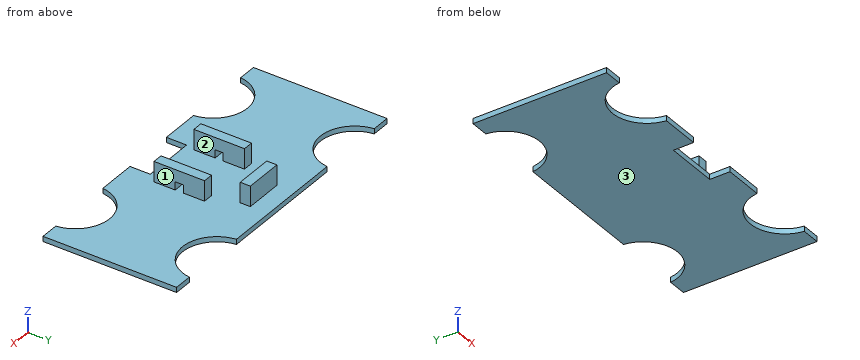
```python
from build123d import *

# Parameters (mm, degrees)
BOSS_EXTRUDE1_DEPTH = 2.54
SKETCH2_W           = 26.0160991
SKETCH2_H           = 10
CUT_EXTRUDE1_DEPTH  = 2.54
SKETCH6_W           = 5
SKETCH6_H           = 25
BOSS_EXTRUDE2_DEPTH = 10
SKETCH6_3_W         = 19
SKETCH6_3_H         = 5
BOSS_EXTRUDE3_DEPTH = 10
SKETCH6_4_W         = 5
SKETCH6_4_H         = 25
BOSS_EXTRUDE4_DEPTH = 10
SKETCH9_W           = 4
SKETCH9_H           = 2
CUT_EXTRUDE3_DEPTH  = 99.671329208


with BuildPart() as part:
    # Sketch1 → Boss-Extrude1 (new body)
    with BuildSketch(Plane.XY):
        with BuildLine():
            Line((-32.468057, 32.999999883), (-13, 32.999999883))
            Line((-13, 32.999999883), (13, 32.999999883))
            Line((13, 32.999999883), (32.468057241, 32.999999883))
            ThreePointArc((32.468057241, 32.999999883), (49.350000777, 18.000000029), (66.231944118, 33.000000103))
            Line((66.231944118, 33.000000103), (75.350000118, 33.000000103))
            Line((75.350000118, 33.000000103), (75.350000118, -32.999998949))
            Line((75.350000118, -32.999998949), (66.231943, -32.999998949))
            ThreePointArc((66.231943, -32.999998949), (49.349999056, -17.999999409), (32.468056, -32.999999949))
            Line((32.468056, -32.999999949), (13, -32.999999949))
            Line((13, -32.999999949), (-12.999999882, -32.999999949))
            Line((-12.999999882, -32.999999949), (-32.468057, -32.999999117))
            ThreePointArc((-32.468057, -32.999999117), (-49.350000944, -17.999999578), (-66.231944, -33.000000117))
            Line((-66.231944, -33.000000117), (-75.35, -33.000000117))
            Line((-75.35, -33.000000117), (-75.35, 32.999999883))
            Line((-75.35, 32.999999883), (-66.231944, 32.999999883))
            ThreePointArc((-66.231944, 32.999999883), (-49.3500005, 17.999999403), (-32.468057, 32.999999883))
        make_face()
    extrude(amount=BOSS_EXTRUDE1_DEPTH)

    # Sketch2 → Cut-Extrude1 (cut)
    with BuildSketch(Plane.XY.offset(2.54)):
        with Locations((0.008049668, -27.999999949)):
            Rectangle(SKETCH2_W, SKETCH2_H)
    extrude(amount=-CUT_EXTRUDE1_DEPTH, mode=Mode.SUBTRACT)

    # Sketch6 → Boss-Extrude2 (add)
    with BuildSketch(Plane.XY.offset(2.54)):
        with Locations((-14.289999882, -6.066775281)):
            Rectangle(SKETCH6_W, SKETCH6_H)
    extrude(amount=BOSS_EXTRUDE2_DEPTH)

    # Sketch6_3 → Boss-Extrude3 (add)
    with BuildSketch(Plane.XY.offset(2.54)):
        with Locations((0.010000118, 21.520000051)):
            Rectangle(SKETCH6_3_W, SKETCH6_3_H)
    extrude(amount=BOSS_EXTRUDE3_DEPTH)

    # Sketch6_4 → Boss-Extrude4 (add)
    with BuildSketch(Plane.XY.offset(2.54)):
        with Locations((14.310000118, -6.066775281)):
            Rectangle(SKETCH6_4_W, SKETCH6_4_H)
    extrude(amount=BOSS_EXTRUDE4_DEPTH)

    # Sketch9 → Cut-Extrude3 (cut, through all)
    with BuildSketch(Plane.ZY.offset(16.789999882)):
        with Locations((4.54, -5.066775281)):
            Rectangle(SKETCH9_W, SKETCH9_H)
        with Locations((4.54, -7.066775281)):
            Rectangle(SKETCH9_W, SKETCH9_H)
    extrude(amount=-CUT_EXTRUDE3_DEPTH, mode=Mode.SUBTRACT)


solid = part.part
```
CAD build for the part. Positions are in the model's coordinates, mm. Face numbers are marked on the shaded views. Coordinates: 2 decimals unless noted, no trailing zeros. Write each loop counter-clockwise with the first axis right and the second up, starting at its lowest first coordinate (ties: lowest second). Pieces come first, ordered by that corner, then holes.
(1) Cut at A-A, the plane z = 10.75. List the corners of the cut face in (x, y), and give its area (3 significant figures).
(2) Two-plate mould, pull along X, no slides. Class the marked faces 1, 2 and 3: +X half, -X half, draft (parallel to the pull), parting line (faces both ways), or undercut.
(3) Cut at D-D, the plane z = 4.5. List the corners of the cut face in (x, y), and give its area (3 significant figures).
(4) Flat gauge pins, fed straight in: pin 1 (1.5 mm diameter, centred on x = -15, z = 7, fed in from -Y); pin 2 (5 mm diameter, centred on y = -5, z = 6, fed in from -X); pin 3 (1.5 mm diameter, centred on x = -8.5, y = -15.5, fed in from +Z). Where does each tip first touch, or does it go through?
(5) Cut at B-B, the plane x = 15. List the corners of the cut face in (y, z), and give its area (3 significant figures).
(6) Drill centre lines: probe 1 along X at (y, z) = (-1, 8.25); probe 2 along Z at (x, y) = (27, -29); probe 3 along X at (y, z) = (22.5, 5.75). Where is each one in solid material? Low to high.
(7) Cut at C-C, the plane y = -15.5. List the corners of the cut face in (x, z).
Geometry says:
1. outline: (-16.79, -18.57) - (-11.79, -18.57) - (-11.79, 6.43) - (-16.79, 6.43) - close; (-9.49, 19.02) - (9.51, 19.02) - (9.51, 24.02) - (-9.49, 24.02) - close; (11.81, -18.57) - (16.81, -18.57) - (16.81, 6.43) - (11.81, 6.43) - close
1. area: 345 mm2
2. face 1: +X half
2. face 2: undercut
2. face 3: draft
3. outline: (-16.79, -18.57) - (-11.79, -18.57) - (-11.79, -8.07) - (-16.79, -8.07) - close; (-16.79, -4.07) - (-11.79, -4.07) - (-11.79, 6.43) - (-16.79, 6.43) - close; (-9.49, 19.02) - (9.51, 19.02) - (9.51, 24.02) - (-9.49, 24.02) - close; (11.81, -18.57) - (16.81, -18.57) - (16.81, -8.07) - (11.81, -8.07) - close; (11.81, -4.07) - (16.81, -4.07) - (16.81, 6.43) - (11.81, 6.43) - close
3. area: 305 mm2
4. pin 1: stops at y = -18.57
4. pin 2: stops at x = -16.79
4. pin 3: stops at z = 2.54
5. outline: (-33, 0) - (33, 0) - (33, 2.54) - (6.43, 2.54) - (6.43, 12.54) - (-18.57, 12.54) - (-18.57, 2.54) - (-33, 2.54) - close; hole (-8.07, 2.54) - (-4.07, 2.54) - (-4.07, 6.54) - (-8.07, 6.54) - close
5. area: 402 mm2
6. probe 1: x = -16.79 to -11.79, 11.81 to 16.81
6. probe 2: z = 0 to 2.54
6. probe 3: x = -9.49 to 9.51
7. outline: (-75.35, 0) - (75.35, 0) - (75.35, 2.54) - (16.81, 2.54) - (16.81, 12.54) - (11.81, 12.54) - (11.81, 2.54) - (-11.79, 2.54) - (-11.79, 12.54) - (-16.79, 12.54) - (-16.79, 2.54) - (-75.35, 2.54) - close
